from build123d import *

# Parameters (mm, degrees)
SKETCH1_R           = 2.1
SKETCH1_R_2         = 10
BOSS_EXTRUDE1_DEPTH = 12.7
SKETCH2_R           = 14.35
CUT_EXTRUDE1_DEPTH  = 8.1
CUT_EXTRUDE2_START  = -12.7
SKETCH3_R           = 14.35
CUT_EXTRUDE2_DEPTH  = 9.1
CUT_EXTRUDE3_START  = -12.7
CUT_EXTRUDE3_DEPTH  = 5
CUT_EXTRUDE4_DEPTH  = 20


with BuildPart() as part:
    # Sketch1 → Boss-Extrude1 (new body)
    with BuildSketch(Plane(origin=(0, 0, 0), x_dir=(1, 0, 0), z_dir=(0, 1, 0))):
        with BuildLine():
            Line((0, 42.5), (-137.9, 42.5))
            ThreePointArc((-137.9, 42.5), (-180.4, 0), (-137.9, -42.5))
            Line((-137.9, -42.5), (0, -42.5))
            ThreePointArc((0, -42.5), (42.5, 0), (0, 42.5))
        make_face()
        with Locations(Location((-102.9, 0, 0), (0, 0, 270))):
            Circle(SKETCH1_R, mode=Mode.SUBTRACT)
        with Locations(Location((-137.9, 35, 0), (0, 0, 270))):
            Circle(SKETCH1_R, mode=Mode.SUBTRACT)
        with Locations(Location((-137.9, -35, 0), (0, 0, 270))):
            Circle(SKETCH1_R, mode=Mode.SUBTRACT)
        with Locations(Location((-172.9, 0, 0), (0, 0, 270))):
            Circle(SKETCH1_R, mode=Mode.SUBTRACT)
        with Locations(Location((-137.9, 0, 0), (0, 0, 270))):
            Circle(SKETCH1_R_2, mode=Mode.SUBTRACT)
        with Locations(Location((0, 35, 0), (0, 0, 270))):
            Circle(SKETCH1_R, mode=Mode.SUBTRACT)
        with Locations(Location((0, -35, 0), (0, 0, 270))):
            Circle(SKETCH1_R, mode=Mode.SUBTRACT)
        with Locations(Location((-17.67766953, -17.67766953, 0), (0, 0, 270))):
            Circle(SKETCH1_R, mode=Mode.SUBTRACT)
        with Locations(Location((17.67766953, -17.67766953, 0), (0, 0, 270))):
            Circle(SKETCH1_R, mode=Mode.SUBTRACT)
        with Locations(Location((-35, 0, 0), (0, 0, 270))):
            Circle(SKETCH1_R, mode=Mode.SUBTRACT)
        with Locations(Location((-17.67766953, 17.67766953, 0), (0, 0, 270))):
            Circle(SKETCH1_R, mode=Mode.SUBTRACT)
        with Locations(Location((0, 0, 0), (0, 0, 270))):
            Circle(SKETCH1_R_2, mode=Mode.SUBTRACT)
        with Locations(Location((35, 0, 0), (0, 0, 270))):
            Circle(SKETCH1_R, mode=Mode.SUBTRACT)
        with Locations(Location((17.67766953, 17.67766953, 0), (0, 0, 270))):
            Circle(SKETCH1_R, mode=Mode.SUBTRACT)
    extrude(amount=-BOSS_EXTRUDE1_DEPTH)

    # Sketch2 → Cut-Extrude1 (cut)
    with BuildSketch(Plane(origin=(0, 0, 0), x_dir=(1, 0, 0), z_dir=(0, 1, 0))):
        with Locations(Location((0, 0, 0), (0, 0, 270))):
            Circle(SKETCH2_R)
    extrude(amount=-CUT_EXTRUDE1_DEPTH, mode=Mode.SUBTRACT)

    # Sketch3 → Cut-Extrude2 (cut)
    with BuildSketch(Plane(origin=(0, 0, 0), x_dir=(1, 0, 0), z_dir=(0, 1, 0)).offset(CUT_EXTRUDE2_START)):
        with Locations(Location((-137.9, 0, 0), (0, 0, 270))):
            Circle(SKETCH3_R)
    extrude(amount=CUT_EXTRUDE2_DEPTH, mode=Mode.SUBTRACT)

    # Sketch4 → Cut-Extrude3 (cut)
    with BuildSketch(Plane(origin=(0, 0, 0), x_dir=(1, 0, 0), z_dir=(0, 1, 0)).offset(CUT_EXTRUDE3_START)):
        with BuildLine():
            Line((-162.9, -4.05), (-172.9, -4.05))
            ThreePointArc((-172.9, -4.05), (-176.95, 0), (-172.9, 4.05))
            Line((-172.9, 4.05), (-162.9, 4.05))
            ThreePointArc((-162.9, 4.05), (-158.85, 0), (-162.9, -4.05))
        make_face()
        with BuildLine():
            Line((-137.9, -30.95), (-127.9, -30.95))
            ThreePointArc((-127.9, -30.95), (-123.85, -35), (-127.9, -39.05))
            Line((-127.9, -39.05), (-137.9, -39.05))
            ThreePointArc((-137.9, -39.05), (-141.95, -35), (-137.9, -30.95))
        make_face()
        with BuildLine():
            Line((-92.9, -4.05), (-102.9, -4.05))
            ThreePointArc((-102.9, -4.05), (-106.95, 0), (-102.9, 4.05))
            Line((-102.9, 4.05), (-92.9, 4.05))
            ThreePointArc((-92.9, 4.05), (-88.85, 0), (-92.9, -4.05))
        make_face()
        with BuildLine():
            Line((-137.9, 39.05), (-127.9, 39.05))
            ThreePointArc((-127.9, 39.05), (-123.85, 35), (-127.9, 30.95))
            Line((-127.9, 30.95), (-137.9, 30.95))
            ThreePointArc((-137.9, 30.95), (-141.95, 35), (-137.9, 39.05))
        make_face()
    extrude(amount=CUT_EXTRUDE3_DEPTH, mode=Mode.SUBTRACT)

    # Sketch6 → Cut-Extrude4 (cut)
    with BuildSketch(Plane(origin=(0, 0, 0), x_dir=(1, 0, 0), z_dir=(0, 1, 0))):
        Polygon((-92.9, 10.860556918), (-52.9, 10.860556918), (-52.9, -10.860556918), (-92.9, -10.860556918), (-92.9, -58.166636569), (47.985280952, -58.166636569), (47.985280952, 58.166636569), (-92.9, 58.166636569), align=None)
    extrude(amount=-CUT_EXTRUDE4_DEPTH, mode=Mode.SUBTRACT)


solid = part.part
Source: CAD feature listing. Evaluate the final solid. Frame: model axes, mm. A direction names the side the tool comes from. Coordinates: 2 decimals unless noted, no trailing zeros. Loops run counter-clockwise (first coordinate to the right, second up) from the corner with the lowest first, then second, coordinate; pieces in that order, holes last. Notation, with made-up numbers: (-24, 19) - (21, 19) arc R10 cw to (21, 37) - close; hole circle Ø5 at (-33.75, -33). An arc over 180 degrees is marked (long way). One line per item, written item: value. Start each with the question number.
1. Section D-D (x = -84.5). Return the cut outline in (y, z).
2. Section B-B (y = -5.75). Return the cut outline in (x, z), and give its area (3 significant figures).
3. Section C-C (x = -144). Return the cut outline in (y, z), and give its area (3 significant figures).
4. Contact query for flat-ended pins moving along their axis: P1, Ø8.5, axis at x = -138, z = 7, coming from the -Y side; P2, Ø4, axis at y = -7, z = -6, coming from the -X side; P3, Ø5, axis at x = -142.5, y = -8.5, coming from the +Z side. Output: stop coordinate, or through.
5. Mould query, pull axis X, two halves, no side actions, for faces 3 (the flat face through (-98, -10, 4.05)), 4 (the flat face through (-73, -6, 10.861)), 5 (the flat face through (-128, -3.6, 3)). Classes: pulls with the +X half, pulls with the -X half, needs draft (parallel to the pull), parting line crosses it, or undercut.
6. Ray query, L1, parallel to X at y = -9.75, z = 0; L2, parallel to X at y = -3.75, z = 0; L3, parallel to Z at x = -135, y = -7.75. Return the intervals inside material, ascending.
7. Section A-A (z = 0). Return the cut outline in (x, y).
8. Set-up query: faces 1 (the cylindrical face through (-140, -4, -35)), 2 (the flat face through (-133, -10, -30.95)). Return all of +Z, -Z, +X, -X, +Y, -Y with unobstructed straight access to the full face (end or side cutting, diameter ignored); none if empty.
Verdict:
1. outline: (-12.7, -10.86) - (0, -10.86) - (0, 10.86) - (-12.7, 10.86) - close
2. outline: (-137.9, -42.5) - (-92.9, -42.5) - (-92.9, -10.86) - (-52.9, -10.86) - (-52.9, 10.86) - (-92.9, 10.86) - (-92.9, 42.5) - (-137.9, 42.5) arc R42.5 ccw to start; hole circle Ø4.2 at (-172.9, 0); hole circle Ø28.7 at (-137.9, 0); hole circle Ø4.2 at (-137.9, -35); hole circle Ø4.2 at (-137.9, 35); hole circle Ø4.2 at (-102.9, 0)
2. area: 6,830 mm2
3. outline: (-12.7, -42.06) - (0, -42.06) - (0, -7.92) - (-3.6, -7.92) - (-3.6, -12.99) - (-12.7, -12.99) - close; (-12.7, 12.99) - (-3.6, 12.99) - (-3.6, 7.92) - (0, 7.92) - (0, 42.06) - (-12.7, 42.06) - close
3. area: 775 mm2
4. P1: stops at y = -3.6
4. P2: stops at x = -180.21
4. P3: stops at z = 42.45
5. face 3: undercut
5. face 4: needs draft
5. face 5: undercut
6. L1: x = -180.4 to -176.95, -158.85 to -152.25, -123.55 to -106.95, -88.85 to -52.9
6. L2: x = -180.4 to -175, -170.8 to -152.25, -123.55 to -105, -100.8 to -52.9
6. L3: z = -42.5 to -39.05, -30.95 to -14.05, 14.05 to 30.95, 39.05 to 42.5
7. outline: (-180.4, -12.7) - (-176.95, -12.7) - (-176.95, -7.7) - (-175, -7.7) - (-175, 0) - (-180.4, 0) - close; (-170.8, -7.7) - (-158.85, -7.7) - (-158.85, -12.7) - (-152.25, -12.7) - (-152.25, -3.6) - (-147.9, -3.6) - (-147.9, 0) - (-170.8, 0) - close; (-127.9, -3.6) - (-123.55, -3.6) - (-123.55, -12.7) - (-106.95, -12.7) - (-106.95, -7.7) - (-105, -7.7) - (-105, 0) - (-127.9, 0) - close; (-100.8, -7.7) - (-88.85, -7.7) - (-88.85, -12.7) - (-52.9, -12.7) - (-52.9, 0) - (-100.8, 0) - close
8. face 1: +Y, -Y
8. face 2: -Y
